from build123d import *

# Parameters (mm, degrees)
CUT_EXTRUDE1_START  = 0.7366
CUT_EXTRUDE1_DEPTH  = 10.922
CIRPATTERN1_COUNT   = 15
FILLET1_R           = 0.381
SKETCH7_R           = 15.0876
BOSS_EXTRUDE1_DEPTH = 12.7
CUT_EXTRUDE3_DEPTH  = 12.7


# Read off the part's stored shape, not the designer's step: Split1
with BuildPart() as part:
    # Sketch2 → Revolve1 (revolve)
    with BuildSketch(Plane(origin=(0, 0, 0), x_dir=(0, 0, -1), z_dir=(1, 0, 0)), mode=Mode.PRIVATE) as revolve1_sk:
        with BuildLine():
            Line((-11.8745, 0), (11.8745, 0))
            Line((11.8745, 0), (11.8745, 15.0876))
            Line((11.8745, 15.0876), (11.02995, 15.0876))
            ThreePointArc((11.02995, 15.0876), (10.408190439, 14.337674152), (10.1854, 13.389339743))
            Line((10.1854, 13.389339743), (10.1854, 11.691079486))
            Line((10.1854, 11.691079486), (-0.7366, 11.691079486))
            Line((-0.7366, 11.691079486), (-0.7366, 13.389339743))
            ThreePointArc((-0.7366, 13.389339743), (-0.959390439, 14.337674152), (-1.58115, 15.0876))
            Line((-1.58115, 15.0876), (-2.4257, 15.0876))
            Line((-2.4257, 15.0876), (-2.4257, 7.9375))
            Line((-2.4257, 7.9375), (-11.8745, 7.9375))
            Line((-11.8745, 7.9375), (-11.8745, 0))
        make_face()
    revolve(revolve1_sk.sketch.rotate(Axis((0, 0, 11.8745), (0, 0, -1)), 90), axis=Axis((0, 0, 11.8745), (0, 0, -1)))

    # Sketch3 → Cut-Extrude1 (cut)
    with BuildSketch(Plane.XY.offset(CUT_EXTRUDE1_START)):
        with BuildLine():
            Line((-0.690489274, 10.3505), (0.690489274, 10.3505))
            Line((0.690489274, 10.3505), (1.2827, 11.6205))
            ThreePointArc((1.2827, 11.6205), (0, 11.691079486), (-1.2827, 11.6205))
            Line((-1.2827, 11.6205), (-0.690489274, 10.3505))
        make_face()
    cut_extrude1 = extrude(amount=-CUT_EXTRUDE1_DEPTH, mode=Mode.SUBTRACT)

    # CirPattern1: Cut-Extrude1 ×15 about axis
    cirpattern1_axis = Axis((0, 0, 0), (0, 0, 1))
    for i in range(1, CIRPATTERN1_COUNT):
        add(cut_extrude1.rotate(cirpattern1_axis, i * 360 / CIRPATTERN1_COUNT), mode=Mode.SUBTRACT)


with BuildPart() as body_2:
    # Split1: the piece on the far side of the plane
    add(part.part)
    split(bisect_by=Plane.XY.offset(2.4257), keep=Keep.BOTTOM)

    # Fillet1
    fillet1_edges = [body_2.edges().sort_by_distance(p)[0] for p in [
        (-15.0876, 0, 2.4257),
    ]]
    fillet(fillet1_edges, radius=FILLET1_R)

    # Sketch7 → Boss-Extrude1 (add)
    with BuildSketch(Plane(origin=(0, 0, -11.8745), x_dir=(-1, 0, 0), z_dir=(0, 0, -1))):
        with Locations(Location((0, 0, 0), (0, 0, 180))):
            Circle(SKETCH7_R)
    extrude(amount=BOSS_EXTRUDE1_DEPTH)

    # Sketch6 → Cut-Extrude3 (cut)
    with BuildSketch(Plane(origin=(0, 0, -11.8745), x_dir=(-1, 0, 0), z_dir=(0, 0, -1))):
        Polygon((-12, 6.92820323), (-12, -6.92820323), (0, -13.856406461), (12, -6.92820323), (12, 6.92820323), (0, 13.856406461), align=None)
    extrude(amount=CUT_EXTRUDE3_DEPTH, mode=Mode.SUBTRACT)


with BuildPart() as part_1:
    add(part.part)

    # Split1
    split(bisect_by=Plane.XY.offset(2.4257), keep=Keep.TOP)


solid = body_2.part
Verification items for the finished model (mm, model axes). A direction names the side the tool comes from. Give positions to 0.01 mm unless a question says otherwise; leave off trailing zeros. Order: outer loops, then holes, each group sorted by start corner. A loop starts at its lowest first (then second) coordinate and runs counter-clockwise, first axis right, second up. Notation, with made-up numbers: M -7,-15 L 43,-15 A36 ccw 43,20 Z; hole C 37,36.5 d7. An arc over 180 degrees is marked long. Answer as a JSON object with one key per item and string values. Group by question number.
1) Mould release check, pull along Z, two halves, no side actions. Record for faces 5 (the face through (0, 0, 2.426)), 6 (the face through (2.41, 11.44, -4.65)), 7 (the face through (6.084, -10.344, -18.136)): released by +Z, released by -Z, zero draft, split by the parting line, or undercut.
2) Depth check by flat-ended pin: pin 1 Ø10 at (y, z) = (-5.5, -13.5) entering from +X; pin 2 Ø1 at (y, z) = (5.5, -20) entering from -X (3 decimals); pin 3 Ø6 at (x, z) = (-3.5, -14) entering from -Y. Enter the tip coordinate at first touch or a pass-through.
3) Cross-section at A-A (z = -22.5). Enter the section's corners in (x, y).
4) Access from +Z, -Z, +X, -X, +Y, -Y to the whole of each face (thin tool, end or side, straight path). Record for faces 1 (the face through (-9.847, 3.189, -4.648)), 2 (the face through (4, 10, 0.737)), 3 (the face through (-2.143, -10.126, -4.648)), 4 (the face through (5.362, 9.628, -4.648)).
5) Scan lines: line 1 along Y through (x, z) = (0, -18.25); line 2 along X through (y, z) = (10, 0.5); line 3 along Z through (x, y) = (-8.5, 8.5). Record each from-to range of solid material in increasing order. Write a range as [from, to].
Result sheet:
{
 "1": {"face 5": "released by +Z", "face 6": "undercut", "face 7": "zero draft"},
 "2": {"pin 1": "stops at x = 15.08", "pin 2": "stops at x = -14.235", "pin 3": "stops at y = -15.08"},
 "3": {"outline": "C 0,0 d30.18; hole M -12,-6.93 L 0,-13.86 L 12,-6.93 L 12,6.93 L 0,13.86 L -12,6.93 Z"},
 "4": {"face 1": "-X", "face 2": "none", "face 3": "-Y", "face 4": "+Y"},
 "5": {"line 1": "y = [-15.09, -13.86], [13.86, 15.09]", "line 2": "x = [-6.06, -5.79], [-3.57, 3.57], [5.79, 6.06]", "line 3": "z = [-11.87, -10.19], [0.74, 2.43]"}
}
